from build123d import *

# Parameters (mm, degrees)
BOSS_EXTRUDE1_DEPTH = 4.445
SKETCH2_W           = 127
SKETCH2_H           = 19.05
BOSS_EXTRUDE2_DEPTH = 3.81
SKETCH3_W           = 16.51
SKETCH3_H           = 3.81
BOSS_EXTRUDE3_DEPTH = 12.7
SKETCH4_R           = 1.5875
CUT_EXTRUDE1_DEPTH  = 78.501223216
WALLS_DEPTH         = 29.21
FILLET5_R           = 2.54
FILLET7_R           = 1.905
FILLET8_R           = 2.159
FILLET9_R           = 1.27


with BuildPart() as part:
    # Sketch1 → Boss-Extrude1 (new body)
    with BuildSketch(Plane(origin=(0, 0, 0), x_dir=(1, 0, 0), z_dir=(0, 1, 0))):
        Polygon((0, -63.5), (0, 63.5), (3.81, 63.5), (38.1, 63.5), (38.1, -63.5), (3.81, -63.5), align=None)
    extrude(amount=BOSS_EXTRUDE1_DEPTH)

    # Sketch2 → Boss-Extrude2 (add)
    with BuildSketch(Plane.ZY):
        with Locations((0, 9.525)):
            Rectangle(SKETCH2_W, SKETCH2_H)
    extrude(amount=-BOSS_EXTRUDE2_DEPTH)

    # Sketch3 → Boss-Extrude3 (add)
    with BuildSketch(Plane.XY.offset(63.5)):
        with Locations((-4.445, 20.955)):
            Rectangle(SKETCH3_W, SKETCH3_H)
    boss_extrude3 = extrude(amount=-BOSS_EXTRUDE3_DEPTH)

    # Mirror1: Boss-Extrude3 across plane
    add(boss_extrude3.mirror(Plane.XY))

    # Sketch4 → Cut-Extrude1 (cut, through all)
    with BuildSketch(Plane(origin=(0, 22.86, 0), x_dir=(1, 0, 0), z_dir=(0, 1, 0))):
        with Locations(Location((-6.35, 57.15, 0), (0, 0, 270))):
            Circle(SKETCH4_R)
        with Locations((-6.35, -57.15)):
            Circle(SKETCH4_R)
    extrude(amount=-CUT_EXTRUDE1_DEPTH, mode=Mode.SUBTRACT)

    # Sketch6 → Walls (add)
    with BuildSketch(Plane(origin=(0, 4.445, 0), x_dir=(1, 0, 0), z_dir=(0, 1, 0))):
        Polygon((3.81, 63.5), (38.1, 63.5), (38.1, -63.5), (3.81, -63.5), (3.81, -60.325), (34.925, -60.325), (34.925, 0), (34.925, 60.325), (3.81, 60.325), align=None)
    extrude(amount=WALLS_DEPTH)

    # Fillet5
    fillet5_edges = [part.edges().sort_by_distance(p)[0] for p in [
        (3.81, 4.445, 0),
        (3.81, 13.6525, 60.325),
        (19.3675, 4.445, -60.325),
        (3.81, 13.6525, -60.325),
        (34.925, 4.445, 0),
        (34.925, 19.05, -60.325),
        (19.3675, 4.445, 60.325),
        (34.925, 19.05, 60.325),
    ]]
    fillet(fillet5_edges, radius=FILLET5_R)

    # Fillet7
    fillet7_edges = [part.edges().sort_by_distance(p)[0] for p in [
        (38.1, 16.8275, -63.5),
        (38.1, 16.8275, 63.5),
        (0, 9.525, 63.5),
        (0, 9.525, -63.5),
    ]]
    fillet(fillet7_edges, radius=FILLET7_R)

    # Fillet8
    fillet8_edges = [part.edges().sort_by_distance(p)[0] for p in [
        (5.08, 22.86, 60.325),
        (5.08, 22.86, -60.325),
        (1.905, 19.05, 50.8),
        (1.905, 19.05, -50.8),
        (3.81, 22.86, -61.9125),
        (3.81, 22.86, 61.9125),
    ]]
    fillet(fillet8_edges, radius=FILLET8_R)

    # Fillet9
    # the kernel refuses this fillet: 1.27 mm, written as the material it adds along each edge
    with BuildSketch(Plane(origin=(0, 19.05, 50.8), x_dir=(-1, 0, 0), z_dir=(0, 0, 1)), Plane(origin=(0, 19.05, -61.595), x_dir=(-1, 0, 0), z_dir=(0, 0, 1))) as fillet9_piece_1:
        with BuildLine():
            CenterArc((FILLET9_R, FILLET9_R), FILLET9_R, 180, 90)
            Line((0, FILLET9_R), (0, 0))
            Line((0, 0), (FILLET9_R, 0))
        make_face()
    extrude(amount=10.795)
    with BuildSketch(Plane(origin=(1.905, 19.05, -61.595), x_dir=(0.995343646445092, 0, 0.09638996566752997), z_dir=(-0.09638996566752997, 0, 0.995343646445092))) as fillet9_piece_2_section:
        with BuildLine():
            CenterArc((1.905 + FILLET9_R, -FILLET9_R), FILLET9_R, 90, 90)
            Line((1.905, -FILLET9_R), (1.905, 0))
            Line((1.905, 0), (1.905 + FILLET9_R, 0))
        make_face()
    fillet9_piece_2 = revolve(axis=Axis((1.905, 19.05, -61.595), (0, 1, 0)), revolution_arc=185.531326158, mode=Mode.PRIVATE)
    fillet9_piece_2 = split(fillet9_piece_2, bisect_by=Plane(origin=(1.905, 19.05, -63.5), z_dir=(0, 0, 1)), keep=Keep.TOP, mode=Mode.PRIVATE)
    add(fillet9_piece_2)
    with BuildSketch(Plane(origin=(1.905, 19.05, 61.595), x_dir=(0.995343646445092, 0, -0.09638996566752997), z_dir=(-0.09638996566752997, 0, -0.995343646445092))) as fillet9_piece_3_section:
        with BuildLine():
            CenterArc((1.905 + FILLET9_R, FILLET9_R), FILLET9_R, 180, 90)
            Line((1.905 + FILLET9_R, 0), (1.905, 0))
            Line((1.905, 0), (1.905, FILLET9_R))
        make_face()
    fillet9_piece_3 = revolve(axis=Axis((1.905, 19.05, 61.595), (0, -1, 0)), revolution_arc=185.531326158, mode=Mode.PRIVATE)
    fillet9_piece_3 = split(fillet9_piece_3, bisect_by=Plane(origin=(1.905, 19.05, 63.5), z_dir=(0, 0, -1)), keep=Keep.TOP, mode=Mode.PRIVATE)
    add(fillet9_piece_3)


solid = part.part
Part model, mm, in its own coordinate system. A direction names the side the tool comes from. Coordinates: 2 decimals unless noted, no trailing zeros. Order: outer loops, then holes, each group sorted by start corner. A loop starts at its lowest first (then second) coordinate and runs counter-clockwise, first axis right, second up. Notation, with made-up numbers: (18, 79) - (53, 79) arc R9 cw to (53, 87) - close; hole circle Ø6 at (45.5, 51.5). An arc over 180 degrees is marked (long way). Use CSV: the item, a comma, the result in double quotes.
Item 1: Saw through at B-B on y = 30.5. Give the cut face in (x, z) (3 decimals).
Solved:
outline,"(3.81, -63.5) - (36.195, -63.5) arc R1.905 ccw to (38.1, -61.595) - (38.1, 61.595) arc R1.905 ccw to (36.195, 63.5) - (3.81, 63.5) - (3.81, 60.325) - (32.385, 60.325) arc R2.54 cw to (34.925, 57.785) - (34.925, -57.785) arc R2.54 cw to (32.385, -60.325) - (3.81, -60.325) - close"
Item 2: Drop flat-ended pins along their axis: P1, Ø1.6, axis at y = 30.5, z = -62, coming from the -X side; P2, Ø3.5, axis at x = -6, z = 56.5, coming from the -Y side; P3, Ø5, axis at x = -4, y = 6.5, coming from the -Z side; P4, Ø21, axis at x = 14, z = 11, coming from the +Y side. Give the stop position or say it passes through.
Solved:
P1,"stops at x = 3.81"
P2,"stops at y = 19.05"
P3,"passes through"
P4,"stops at y = 19.05"
Item 3: Mould opens along X. For faces 4 (the face through (-6, 21, 50.8)), 5 (the face through (4.534, 16.128, -59.561)), 6 (the face through (-12.7, 21, -57)), 7 (the face through (18, 20, -60.325)) say: +X half, -X half, draft (parallel to the pull), parting line (faces both ways), or undercut.
Solved:
face 4,"draft"
face 5,"undercut"
face 6,"-X half"
face 7,"undercut"
Item 4: 3-axis set-ups, long thin cutter, end or side, ignore diameter. For faces 1 (the face through (2, 19.05, -1)), 2 (the face through (-6.7, 21, 58.7)), 3 (the face through (34.2, 20.51, 59.56)): which of +Z, -Z, +X, -X, +Y, -Y reach the whole face in a straight line?
Solved:
face 1,"-X, +Y"
face 2,"+Y, -Y"
face 3,"+Y"
Item 5: Probe probe 1 along X at (y, z) = (21.8, 57.15) (1 decimal); probe 2 along Z at (x, y) = (16, 29.5) (3 decimals); probe 3 along X at (y, z) = (15, 31.5) (3 decimals). List the from-to ranges inside material, lowest first.
Solved:
probe 1,"x = -12.7 to -7.9, -4.8 to 3.8, 34.9 to 38.1"
probe 2,"z = -63.5 to -60.325, 60.325 to 63.5"
probe 3,"x = 0 to 3.81, 34.925 to 38.1"
Item 6: Saw through at D-D on x = -6.35. Give the cut face in (y, z), and give its area (3 significant figures).
Solved:
outline,"(19.05, -63.5) - (22.86, -63.5) - (22.86, -58.74) - (19.05, -58.74) - close; (19.05, -55.56) - (22.86, -55.56) - (22.86, -50.8) - (19.05, -50.8) - close; (19.05, 50.8) - (22.86, 50.8) - (22.86, 55.56) - (19.05, 55.56) - close; (19.05, 58.74) - (22.86, 58.74) - (22.86, 63.5) - (19.05, 63.5) - close"
area,"72.6 mm²"
Item 7: Saw through at C-C on z = 26.5. Give the cut face in (x, y) (3 decimals).
Solved:
outline,"(0, 0) - (38.1, 0) - (38.1, 33.655) - (34.925, 33.655) - (34.925, 6.985) arc R2.54 cw to (32.385, 4.445) - (6.35, 4.445) arc R2.54 cw to (3.81, 6.985) - (3.81, 19.05) - (0, 19.05) - close"
Item 8: Saw through at A-A on x = 9. Give the cut face in (y, z) (3 decimals).
Solved:
outline,"(0, -63.5) - (33.655, -63.5) - (33.655, -60.325) - (6.985, -60.325) arc R2.54 cw to (4.445, -57.785) - (4.445, 57.785) arc R2.54 cw to (6.985, 60.325) - (33.655, 60.325) - (33.655, 63.5) - (0, 63.5) - close"
